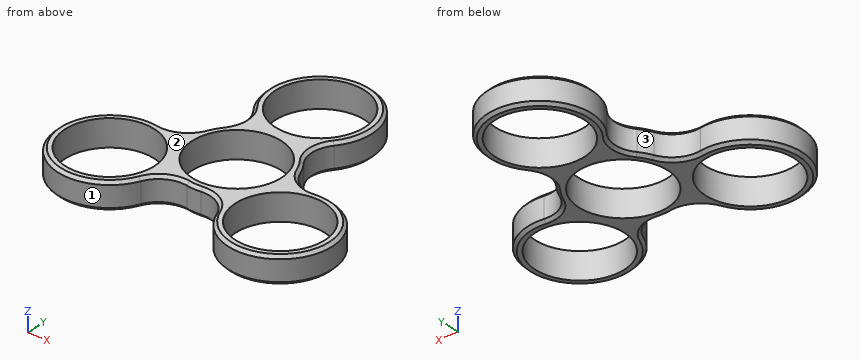
from build123d import *

# Parameters (mm, degrees)
F0_R      = 17.5
F1_DEPTH  = 9
F2_R      = 17.5
F3_DEPTH  = 9
F4_R      = 15
F6_DEPTH  = 25
F5_R      = 15
F7_DEPTH  = 25
F8_R      = 15
F9_DEPTH  = 25
F10_R     = 15
F11_DEPTH = 25
F12_R     = 10
F13_SIZE  = 1
F14_SIZE  = 1


with BuildPart() as f1:
    # F0 (on Top) → F1 (new body)
    with BuildSketch(Plane.XY):
        Circle(F0_R)
    extrude(amount=F1_DEPTH)

    # F2 (on Top) → F3 (join)
    with BuildSketch(Plane.XY):
        with Locations((0, 33.7313876416)):
            Circle(F2_R)
        with Locations((29.2122386025, -16.8656938208)):
            Circle(F2_R)
        with Locations((-29.2122386025, -16.8656938208)):
            Circle(F2_R)
    extrude(amount=F3_DEPTH)

    # F4 (on face) → F6 (cut)
    with BuildSketch(Plane(origin=(0, 0, 0), x_dir=(1, 0, 0), z_dir=(0, 0, -1))):
        with Locations((0, -33.7313876416)):
            Circle(F4_R)
    extrude(amount=-F6_DEPTH, mode=Mode.SUBTRACT)

    # F5 (on face) → F7 (cut)
    with BuildSketch(Plane(origin=(0, 0, 0), x_dir=(1, 0, 0), z_dir=(0, 0, -1))):
        Circle(F5_R)
    extrude(amount=-F7_DEPTH, mode=Mode.SUBTRACT)

    # F8 (on face) → F9 (cut)
    with BuildSketch(Plane(origin=(0, 0, 0), x_dir=(1, 0, 0), z_dir=(0, 0, -1))):
        with Locations((-29.2122386025, 16.8656938208)):
            Circle(F8_R)
    extrude(amount=-F9_DEPTH, mode=Mode.SUBTRACT)

    # F10 (on face) → F11 (cut)
    with BuildSketch(Plane(origin=(0, 0, 0), x_dir=(1, 0, 0), z_dir=(0, 0, -1))):
        with Locations((29.2122386025, 16.8656938208)):
            Circle(F10_R)
    extrude(amount=-F11_DEPTH, mode=Mode.SUBTRACT)

    # F12
    f12_edges = [f1.edges().sort_by_distance(p)[0] for p in [
        (16.940556, -4.389485, 4.5),
        (12.271683, -12.476209, 4.5),
        (-16.940556, -4.389485, 4.5),
        (-12.271683, -12.476209, 4.5),
        (4.668873, 16.865694, 4.5),
        (-4.668873, 16.865694, 4.5),
    ]]
    fillet(f12_edges, radius=F12_R)

    # F13
    f13_edges = [f1.edges().sort_by_distance(p)[0] for p in [
        (44.367683, -25.615694, 0),
    ]]
    chamfer(f13_edges, length=F13_SIZE)

    # F14
    f14_edges = [f1.edges().sort_by_distance(p)[0] for p in [
        (44.367683, -25.615694, 9),
    ]]
    chamfer(f14_edges, length=F14_SIZE)


solid = f1.part
Read the model definition and answer for the solid it produces. Units are mm, in the model's axes. Face numbers are marked on the shaded views. Round coordinates to 2 decimals unless told otherwise and drop trailing zeros. Write each loop counter-clockwise with the first axis right and the second up, starting at its lowest first coordinate (ties: lowest second). Pieces come first, ordered by that corner, then holes. Notation, with made-up numbers: M 50.5,-25 L 106.5,-25 A29 ccw 106.5,6 Z; hole C -2,76.25 d11. An arc over 180 degrees is marked long. Use a Markdown table: item, result.
1) The part is cut by section B-B (y = -13.5). Give the number of separate pieces and of enclosed holes in the cut face, plus the area to 3 significant figures.
Answers follow:
| item | result |
|---|---|
| separate pieces | 4 |
| enclosed holes | 0 |
| area | 189 mm2 |
2) The part is cut by section A-A (x = 0). Write down the section's boundary in (y, z), plus the area to 3 significant figures.
Answers follow:
| item | result |
|---|---|
| outline | M -17.5,1 L -16.5,0 L -15,0 L -15,9 L -16.5,9 L -17.5,8 Z; M 15,0 L 18.73,0 L 18.73,9 L 15,9 Z; M 48.73,0 L 50.23,0 L 51.23,1 L 51.23,8 L 50.23,9 L 48.73,9 Z |
| area | 76.6 mm2 |
3) Straight lines are drawn through the part: line 1 along Y through (x, z) = (0, 4); line 2 along Y through (x, z) = (10.5, 6); line 3 along X through (y, z) = (-13.5, 7.5). For each, find the intervals that lie inside material, in ascending order. Write a range as [from, to].
Answers follow:
| item | result |
|---|---|
| line 1 | y = [-17.5, -15], [15, 18.73], [48.73, 51.23] |
| line 2 | y = [-19.87, -10.71], [10.71, 23.02], [44.44, 47.73] |
| line 3 | x = [-46.39, -43.83], [-14.59, -6.54], [6.54, 14.59], [43.83, 46.39] |
4) For a pull along Y with two mould halves and no side action, classify the marked faces 1, 2 and 3 as pulls with the +Y half, pulls with the -Y half, needs draft (parallel to the pull), parting line crosses it, or undercut.
Answers follow:
| item | result |
|---|---|
| face 1 | parting line crosses it |
| face 2 | needs draft |
| face 3 | undercut |
5) Flat-ended cylindrical pins translate along their axes: pin 1 (3 mm diameter, centred on x = 10.5, z = 3.5, fed in from +Y); pin 2 (1 mm diameter, centred on x = 17.5, y = -2, fed in from -Z); pin 3 (1.5 mm diameter, centred on y = 8.5, z = 2.5, fed in from -X); pin 4 (1 mm diameter, centred on x = -4.5, z = 5, fed in from +Y). Find the tip coordinate at first contact, or state that the pin passes through.
Answers follow:
| item | result |
|---|---|
| pin 1 | stops at y = 48.74 |
| pin 2 | stops at z = 0 |
| pin 3 | stops at x = -15.69 |
| pin 4 | stops at y = 50.77 |
